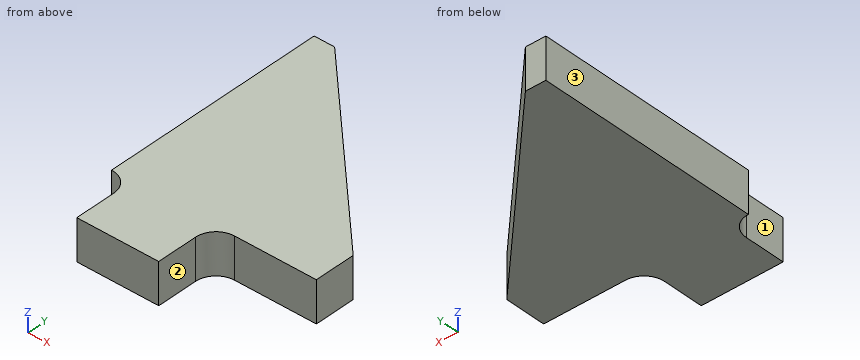
from build123d import *

# Parameters (mm, degrees)
BOSS_EXTRU_1_DEPTH = 2
CONG_1_R           = 1


with BuildPart() as part:
    # Esquisse1 → Boss.-Extru.1 (new body)
    with BuildSketch(Plane.XY):
        Polygon((0, 0), (0, 11), (1, 11), (10, 2), (10, 0), (5, 0), (5, -3), (1, -3), (1, 0), align=None)
    extrude(amount=BOSS_EXTRU_1_DEPTH)

    # Congé1
    cong_1_edges = [part.edges().sort_by_distance(p)[0] for p in [
        (5, 0, 1),
        (1, 0, 1),
    ]]
    fillet(cong_1_edges, radius=CONG_1_R - 0.0001)  # a hair under: the kernel refuses the full size


solid = part.part
For this review, take the finished solid that the model builds, in its own axes (mm). Face numbers are marked on the shaded views. A direction names the side the tool comes from. Round coordinates to 2 decimals unless told otherwise and drop trailing zeros. Write each loop counter-clockwise with the first axis right and the second up, starting at its lowest first coordinate (ties: lowest second). Pieces come first, ordered by that corner, then holes. Notation, with made-up numbers: (16, 69) - (58, 69) arc R14 ccw to (58, 73) - close; hole circle Ø8 at (13.25, 54). An arc over 180 degrees is marked (long way). Use a Markdown table: item, result.
Q1. Machinability: for the marked faces 1, 2 and 3, which of the approach directions +Z, -Z, +X, -X, +Y, -Y give a long, thin tool a straight path to every point of the face, cutting with its end or side? Answer none if there is none.
Derived:
| item | result |
|---|---|
| face 1 | +Z, -Z, -X, -Y |
| face 2 | +Z, -Z, +X, -Y |
| face 3 | +Z, -Z, -X, +Y, -Y |
Q2. We need section C-C (x = 4.25). Give the boundary of the cut face in (y, z).
Derived:
| item | result |
|---|---|
| outline | (-3, 0) - (7.75, 0) - (7.75, 2) - (-3, 2) - close |
Q3. We need section B-B (y = 5.75). Give the boundary of the cut face in (x, z), plus the area to 3 significant figures.
Derived:
| item | result |
|---|---|
| outline | (0, 0) - (6.25, 0) - (6.25, 2) - (0, 2) - close |
| area | 12.5 mm2 |
Q4. Clearance check with flat-ended pins moving along their axes: pin 1 (1 mm diameter, centred on y = -2, z = 1, fed in from +X); pin 2 (5 mm diameter, centred on x = 8, y = 8.5, fed in from +Z); pin 3 (0.6 mm diameter, centred on y = -1.5, z = 1, fed in from -X); pin 4 (1 mm diameter, centred on x = 7, z = 1, fed in from -Y). State where each tip first meets the part, or that it passes through.
Derived:
| item | result |
|---|---|
| pin 1 | stops at x = 5 |
| pin 2 | passes through |
| pin 3 | stops at x = 1 |
| pin 4 | stops at y = 0 |
Q5. Wall thickness on line 1 along Y through (x, z) = (2, 0.95); line 2 along X through (y, z) = (-2.5, 1.1); line 3 along Y through (x, z) = (5.75, 0.2): over which ranges is each line inside the solid? List them lowest first.
Derived:
| item | result |
|---|---|
| line 1 | y = -3 to 10 |
| line 2 | x = 1 to 5 |
| line 3 | y = -0.03 to 6.25 |
